```python
from build123d import *

# Parameters (mm, degrees)
SKIZZE3_W                          = 330
SKIZZE3_H                          = 100
BASIS_BLECH1_DEPTH                 = 2
KANTE_LASCHE1_STRIP_W              = 8.2
KANTE_LASCHE1_STRIP_H              = 2
KANTE_LASCHE1_STRIP_CUT_DEPTH      = 330
KANTE_LASCHE1_STRIP_2_W            = 8.2
KANTE_LASCHE1_STRIP_2_H            = 2
KANTE_LASCHE1_STRIP_CUT_2_DEPTH    = 330
KANTE_LASCHE1_DEPTH                = 330
KANTE_LASCHE1_BEND_DEPTH           = 330
KANTE_LASCHE5_DEPTH                = 99.8
KANTE_LASCHE5_BEND_DEPTH           = 99.8
KANTE_LASCHE3_STRIP_W              = 8.2
KANTE_LASCHE3_STRIP_H              = 2
KANTE_LASCHE3_STRIP_CUT_DEPTH      = 330
KANTE_LASCHE3_STRIP_2_W            = 8.2
KANTE_LASCHE3_STRIP_2_H            = 2
KANTE_LASCHE3_STRIP_CUT_2_DEPTH    = 330
KANTE_LASCHE3_DEPTH                = 330
KANTE_LASCHE3_BEND_DEPTH           = 330
VERRUNDUNG2_R                      = 10
F_5_0_5_DURCHMESSER_BOHRUNG1_D     = 5
F_5_0_5_DURCHMESSER_BOHRUNG1_DEPTH = 10
F_5_0_5_DURCHMESSER_BOHRUNG1_TIP   = 1.502151548
GESCHLOSSENE_START                 = -52
GESCHLOSSENE_ECKE2_OUTLINE_W       = 2
GESCHLOSSENE_ECKE2_OUTLINE_H       = 79.9
GESCHLOSSENE_ECKE2_DEPTH           = 2.1
GESCHLOSSENE_START_2               = 49.9
GESCHLOSSENE_ECKE2_2_OUTLINE_W     = 2
GESCHLOSSENE_ECKE2_2_OUTLINE_H     = 79.9
GESCHLOSSENE_ECKE2_2_DEPTH         = 2.1


# Read off the part's stored shape, not the designer's step: Geschlossene Ecke2
# Sheet-metal steps are written as plain solids
with BuildPart() as part:
    # Skizze3 → Basis-Blech1 (new body)
    with BuildSketch(Plane(origin=(0, 0, 0), x_dir=(1, 0, 0), z_dir=(0, 1, 0))):
        Rectangle(SKIZZE3_W, SKIZZE3_H)
    extrude(amount=-BASIS_BLECH1_DEPTH)

    # Kante-Lasche1 strip (across the edge) → Kante-Lasche1 strip cut (cut)
    with BuildSketch(Plane(origin=(-165, -2, -50), x_dir=(0, 0, 1), z_dir=(1, 0, 0))):
        with Locations((-4, -1)):
            Rectangle(KANTE_LASCHE1_STRIP_W, KANTE_LASCHE1_STRIP_H)
    extrude(amount=KANTE_LASCHE1_STRIP_CUT_DEPTH, mode=Mode.SUBTRACT)

    # Kante-Lasche1 strip 2 (across the edge) → Kante-Lasche1 strip cut 2 (cut)
    with BuildSketch(Plane(origin=(165, -2, 50), x_dir=(0, 0, -1), z_dir=(-1, 0, 0))):
        with Locations((-4, -1)):
            Rectangle(KANTE_LASCHE1_STRIP_2_W, KANTE_LASCHE1_STRIP_2_H)
    extrude(amount=KANTE_LASCHE1_STRIP_CUT_2_DEPTH, mode=Mode.SUBTRACT)

    # Kante-Lasche1 section (across the edge) → Kante-Lasche1 (add)
    with BuildSketch(Plane(origin=(-165, -2, -50), x_dir=(0, 0, 1), z_dir=(1, 0, 0))):
        with BuildLine():
            Line((-2, 0.1), (-2, 80))
            Line((-2, 80), (0, 80))
            Line((0, 80), (0, 0.1))
            ThreePointArc((0, 0.1), (0.029289322, 0.029289322), (0.1, 0))
            Line((0.1, 0), (0.1, -2))
            ThreePointArc((0.1, -2), (-1.38492424, -1.38492424), (-2, 0.1))
        make_face()
    extrude(amount=KANTE_LASCHE1_DEPTH)

    # Kante-Lasche1 section 2 (across the edge) → Kante-Lasche1 bend (add)
    with BuildSketch(Plane(origin=(165, -2, 50), x_dir=(0, 0, -1), z_dir=(-1, 0, 0))):
        with BuildLine():
            Line((-2, 0.1), (-2, 80))
            Line((-2, 80), (0, 80))
            Line((0, 80), (0, 0.1))
            ThreePointArc((0, 0.1), (0.029289322, 0.029289322), (0.1, 0))
            Line((0.1, 0), (0.1, -2))
            ThreePointArc((0.1, -2), (-1.38492424, -1.38492424), (-2, 0.1))
        make_face()
    extrude(amount=KANTE_LASCHE1_BEND_DEPTH)

    # Kante-Lasche5 section (across the edge) → Kante-Lasche5 (add)
    with BuildSketch(Plane(origin=(-165.1, -2, 49.9), x_dir=(1, 0, 0), z_dir=(0, 0, -1))):
        with BuildLine():
            Line((-2, 0.1), (-2, 80))
            Line((-2, 80), (0, 80))
            Line((0, 80), (0, 0.1))
            ThreePointArc((0, 0.1), (0.029289322, 0.029289322), (0.1, 0))
            Line((0.1, 0), (0.1, -2))
            ThreePointArc((0.1, -2), (-1.38492424, -1.38492424), (-2, 0.1))
        make_face()
    extrude(amount=KANTE_LASCHE5_DEPTH)

    # Kante-Lasche5 section 2 (across the edge) → Kante-Lasche5 bend (add)
    with BuildSketch(Plane(origin=(165.1, -2, -49.9), x_dir=(-1, 0, 0), z_dir=(0, 0, 1))):
        with BuildLine():
            Line((-2, 0.1), (-2, 80))
            Line((-2, 80), (0, 80))
            Line((0, 80), (0, 0.1))
            ThreePointArc((0, 0.1), (0.029289322, 0.029289322), (0.1, 0))
            Line((0.1, 0), (0.1, -2))
            ThreePointArc((0.1, -2), (-1.38492424, -1.38492424), (-2, 0.1))
        make_face()
    extrude(amount=KANTE_LASCHE5_BEND_DEPTH)

    # Kante-Lasche3 strip (across the edge) → Kante-Lasche3 strip cut (cut)
    with BuildSketch(Plane(origin=(-165, -82, 52), x_dir=(0, 1, 0), z_dir=(1, 0, 0))):
        with Locations((-2, -1)):
            Rectangle(KANTE_LASCHE3_STRIP_W, KANTE_LASCHE3_STRIP_H)
    extrude(amount=KANTE_LASCHE3_STRIP_CUT_DEPTH, mode=Mode.SUBTRACT)

    # Kante-Lasche3 strip 2 (across the edge) → Kante-Lasche3 strip cut 2 (cut)
    with BuildSketch(Plane(origin=(165, -82, -52), x_dir=(0, 1, 0), z_dir=(-1, 0, 0))):
        with Locations((-2, -1)):
            Rectangle(KANTE_LASCHE3_STRIP_2_W, KANTE_LASCHE3_STRIP_2_H)
    extrude(amount=KANTE_LASCHE3_STRIP_CUT_2_DEPTH, mode=Mode.SUBTRACT)

    # Kante-Lasche3 section (across the edge) → Kante-Lasche3 (add)
    with BuildSketch(Plane(origin=(-165, -82, 52), x_dir=(0, 1, 0), z_dir=(1, 0, 0))):
        with BuildLine():
            Line((0, 0.1), (0, 13))
            Line((0, 13), (2, 13))
            Line((2, 13), (2, 0.1))
            ThreePointArc((2, 0.1), (2.029289322, 0.029289322), (2.1, 0))
            Line((2.1, 0), (2.1, -2))
            ThreePointArc((2.1, -2), (0.61507576, -1.38492424), (0, 0.1))
        make_face()
    extrude(amount=KANTE_LASCHE3_DEPTH)

    # Kante-Lasche3 section 2 (across the edge) → Kante-Lasche3 bend (add)
    with BuildSketch(Plane(origin=(165, -82, -52), x_dir=(0, 1, 0), z_dir=(-1, 0, 0))):
        with BuildLine():
            Line((0, 0.1), (0, 13))
            Line((0, 13), (2, 13))
            Line((2, 13), (2, 0.1))
            ThreePointArc((2, 0.1), (2.029289322, 0.029289322), (2.1, 0))
            Line((2.1, 0), (2.1, -2))
            ThreePointArc((2.1, -2), (0.61507576, -1.38492424), (0, 0.1))
        make_face()
    extrude(amount=KANTE_LASCHE3_BEND_DEPTH)

    # Verrundung2
    verrundung2_edges = [part.edges().sort_by_distance(p)[0] for p in [
        (-165, -81, 65),
        (165, -81, 65),
        (165, -81, -65),
        (-165, -81, -65),
    ]]
    fillet(verrundung2_edges, radius=VERRUNDUNG2_R)

    # Ø5.0 (5) Durchmesser Bohrung1
    with Locations(Plane.ZY.offset(167.1)):
        with Locations((32, -41), (-32, -41)):
            Hole(F_5_0_5_DURCHMESSER_BOHRUNG1_D / 2, depth=F_5_0_5_DURCHMESSER_BOHRUNG1_DEPTH)
            with Locations((0, 0, -(F_5_0_5_DURCHMESSER_BOHRUNG1_DEPTH + F_5_0_5_DURCHMESSER_BOHRUNG1_TIP / 2))):  # 118° drill point
                Cone(0, F_5_0_5_DURCHMESSER_BOHRUNG1_D / 2, F_5_0_5_DURCHMESSER_BOHRUNG1_TIP, mode=Mode.SUBTRACT)

    # Geschlossene Ecke2 outline → Geschlossene Ecke2 (add)
    with BuildSketch(Plane.XY.offset(GESCHLOSSENE_START)):
        with Locations((-166.1, -42.05)):
            Rectangle(GESCHLOSSENE_ECKE2_OUTLINE_W, GESCHLOSSENE_ECKE2_OUTLINE_H)
        with Locations((166.1, -42.05)):
            Rectangle(GESCHLOSSENE_ECKE2_OUTLINE_W, GESCHLOSSENE_ECKE2_OUTLINE_H)
    extrude(amount=GESCHLOSSENE_ECKE2_DEPTH)

    # Geschlossene Ecke2 2 outline → Geschlossene Ecke2 2 (add)
    with BuildSketch(Plane.XY.offset(GESCHLOSSENE_START_2)):
        with Locations((-166.1, -42.05)):
            Rectangle(GESCHLOSSENE_ECKE2_2_OUTLINE_W, GESCHLOSSENE_ECKE2_2_OUTLINE_H)
        with Locations((166.1, -42.05)):
            Rectangle(GESCHLOSSENE_ECKE2_2_OUTLINE_W, GESCHLOSSENE_ECKE2_2_OUTLINE_H)
    extrude(amount=GESCHLOSSENE_ECKE2_2_DEPTH)


solid = part.part
```
Check sheet for the modelled part. Datum: model origin and axes. Units: mm. A direction names the side the tool comes from. Give positions to 0.01 mm unless a question says otherwise; leave off trailing zeros. Loops run counter-clockwise (first coordinate to the right, second up) from the corner with the lowest first, then second, coordinate; pieces in that order, holes last. Notation, with made-up numbers: M 55,6 L 86,6 A23 ccw 86,27 Z; hole C -13,85 d10. An arc over 180 degrees is marked long. Answer in a Markdown table with one row per item.
1) Cross-section at C-C (x = 98). Enter the section's corners in (y, z).
Solutions:
| item | result |
|---|---|
| outline | M -82,-65 L -80,-65 L -80,-52.1 A0.1 cw -79.9,-52 L -2.1,-52 A2.1 ccw 0,-49.9 L 0,49.9 A2.1 ccw -2.1,52 L -79.9,52 A0.1 cw -80,52.1 L -80,65 L -82,65 L -82,52.1 A2.1 ccw -79.9,50 L -2.1,50 A0.1 cw -2,49.9 L -2,-49.9 A0.1 cw -2.1,-50 L -79.9,-50 A2.1 ccw -82,-52.1 Z |
2) Tool access check on faces 1 (the face through (2, -40, 52)), 2 (the face through (-2, -40, -52)), 3 (the face through (2, -42, 50)). Record the directions out of +Z, -Z, +X, -X, +Y, -Y that give a thin tool (end or side, any length) a straight path to the whole face; none if there is none.
Solutions:
| item | result |
|---|---|
| face 1 | +Z, +X, -X, +Y |
| face 2 | -Z, +X, -X, +Y |
| face 3 | -Y |
3) Mould release check, pull along Z, two halves, no side actions. Record for faces 4 (the face through (167.1, -41, -1)), 5 (the face through (162.15, -80.99, 61.99)), 6 (the face through (-2, -42, -50)): released by +Z, released by -Z, zero draft, split by the parting line, or undercut.
Solutions:
| item | result |
|---|---|
| face 4 | zero draft |
| face 5 | released by +Z |
| face 6 | undercut |
4) Cross-section at A-A (y = -47). Enter the section's corners in (x, z).
Solutions:
| item | result |
|---|---|
| outline | M -167.1,-52 L -165.1,-52 L -165.1,52 L -167.1,52 Z; M -165,-52 L 165,-52 L 165,-50 L -165,-50 Z; M -165,50 L 165,50 L 165,52 L -165,52 Z; M 165.1,-52 L 167.1,-52 L 167.1,52 L 165.1,52 Z |
5) Thickness scan on line 1 (X direction, y = -50.5, z = 19); line 2 (Z direction, x = -102, y = -49); line 3 (Y direction, x = -165, z = 32). Record the ranges inside material, lowest first.
Solutions:
| item | result |
|---|---|
| line 1 | x = -167.1 to -165.1, 165.1 to 167.1 |
| line 2 | z = -52 to -50, 50 to 52 |
| line 3 | y = -2 to 0 |
6) Depth check by flat-ended pin: pin 1 (0.6 mm diameter, centred on x = 166, z = -51.5, fed in from +Y); pin 2 (10 mm diameter, centred on x = -111.5, y = -70, fed in from +Z); pin 3 (3 mm diameter, centred on x = 126, z = -6.5, fed in from -Y); pin 4 (1.5 mm diameter, centred on y = -48, z = -53.5, fed in from -X). Enter the tip coordinate at first touch or a pass-through.
Solutions:
| item | result |
|---|---|
| pin 1 | stops at y = -2.1 |
| pin 2 | stops at z = 52 |
| pin 3 | stops at y = -2 |
| pin 4 | passes through |
7) Cross-section at B-B (z = 5.5). Enter the section's corners in (x, y).
Solutions:
| item | result |
|---|---|
| outline | M -167.1,-82 L -165.1,-82 L -165.1,-2.1 A0.1 cw -165,-2 L 165,-2 A0.1 cw 165.1,-2.1 L 165.1,-82 L 167.1,-82 L 167.1,-2.1 A2.1 ccw 165,0 L -165,0 A2.1 ccw -167.1,-2.1 Z |
